Job drawing, mm, ordinate dimensions from the low corner. One solid piece. A direction names the side the tool comes from. Give positions to 0.01 mm unless a question says otherwise; leave off trailing zeros. Order: outer loops, then holes, each group sorted by start corner. A loop starts at its lowest first (then second) coordinate and runs counter-clockwise, first axis right, second up.
Item 1: Band-saw the part on B-B on z = 4.25. Give the cut face in (x, y).
Item 2: Flat gauge pins, fed straight in: P1, Ø2.5, axis at y = 2.5, z = 6.5, coming from the -X side; P2, Ø10, axis at x = 17, y = 9.5, coming from the -Z side; P3, Ø5, axis at y = 9.5, z = 6, coming from the -X side; P4, Ø8, axis at x = 52, y = 17, coming from the +Z side. Where does each tip first touch, or does it go through?
Item 3: Band-saw the part on D-D on x = 15.5. Give the cut face in (y, z).
Item 4: Wall check: L1, parallel to Y at x = 51.5, z = 3.25; L2, parallel to X at y = 17, z = 1; L3, parallel to X at y = 8, z = 5.25. Give the ranges that are in metal, low to high.
Item 5: Band-saw the part on C-C on y = 2.75. Give the cut face in (x, z), plus the area to 3 significant figures.
Item 6: Band-saw the part on A-A on x = 53. Give the cut face in (y, z).
Item 7: Which spindle directions (+Z, -Z, +X, -X, +Y, -Y) get a long thin tool onto all of the face, cutting with end or side? Do the marked faces 1, 2 and 3. Say none if no direction does.
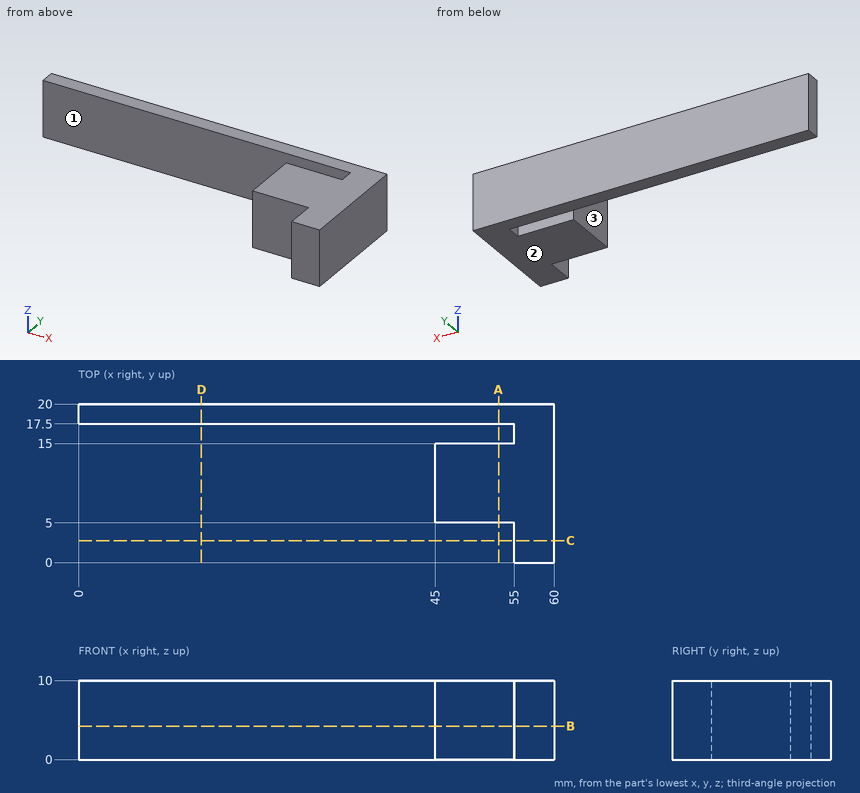
The answers:
1. outline: (0, 17.5) - (55, 17.5) - (55, 15) - (45, 15) - (45, 5) - (55, 5) - (55, 0) - (60, 0) - (60, 20) - (0, 20) - close
2. P1: stops at x = 55
2. P2: passes through
2. P3: stops at x = 45
2. P4: stops at z = 10
3. outline: (17.5, 0) - (20, 0) - (20, 10) - (17.5, 10) - close
4. L1: y = 5 to 15, 17.5 to 20
4. L2: x = 55 to 60
4. L3: x = 45 to 60
5. outline: (55, 0) - (60, 0) - (60, 10) - (55, 10) - close
5. area: 50.0 mm2
6. outline: (5, 0) - (15, 0) - (15, 10) - (5, 10) - close; (17.5, 0) - (20, 0) - (20, 10) - (17.5, 10) - close
7. face 1: +Z, -Z, -X
7. face 2: -Z, +X, -X, +Y, -Y
7. face 3: +Z, -Z, -X, -Y
